```python
from build123d import *
from build123d.topology import SkipClean

# Parameters (mm, degrees)
EXTRUSION1_DEPTH = 20
ESQUISSE2_R      = 3.5
EXTRUSION2_DEPTH = 8
EXTRUSION3_START = -3
EXTRUSION3_DEPTH = 3


with BuildPart() as part:
    # Esquisse1 → Extrusion1 (new body)
    with BuildSketch(Plane.XY):
        Polygon((-21.808080808, -11.643556434), (-21.808080808, 14.356443566), (-28.808080808, 14.356443566), (-28.808080808, 16.356443566), (-21.808080808, 16.356443566), (-21.808080808, 23.356443566), (18.191919192, 23.356443566), (18.191919192, 16.356443566), (25.191919192, 16.356443566), (25.191919192, 14.356443566), (18.191919192, 14.356443566), (18.191919192, -11.643556434), align=None)
    extrude(amount=EXTRUSION1_DEPTH)

    # Esquisse2 → Extrusion2 (add)
    with BuildSketch(Plane(origin=(0, 23.356443566, 0), x_dir=(1, 0, 0), z_dir=(0, 1, 0))):
        with Locations((8.191919192, -10)):
            Circle(ESQUISSE2_R)
    extrude(amount=EXTRUSION2_DEPTH)

    # Esquisse3 → Extrusion3 (add)
    with SkipClean():  # the faces are left unmerged after this step: merging them gives an invalid solid
        with BuildSketch(Plane(origin=(0, 31.356443566, 0), x_dir=(1, 0, 0), z_dir=(0, 1, 0)).offset(EXTRUSION3_START)):
            with BuildLine():
                Line((4.746696028, -9.383203961), (-5.515585224, 0.879077291))
                ThreePointArc((-5.515585224, 0.879077291), (-4.182449479, 2.374368671), (-2.687158099, 3.707504416))
                Line((-2.687158099, 3.707504416), (7.575123153, -6.554776836))
                ThreePointArc((7.575123153, -6.554776836), (8.191919192, -6.5), (8.808715231, -6.554776836))
                Line((8.808715231, -6.554776836), (19.069778625, 3.706286557))
                ThreePointArc((19.069778625, 3.706286557), (20.565077985, 2.373158793), (21.898205749, 0.877859433))
                Line((21.898205749, 0.877859433), (11.637142355, -9.383203961))
                ThreePointArc((11.637142355, -9.383203961), (11.691919192, -10), (11.637142355, -10.616796039))
                Line((11.637142355, -10.616796039), (21.899423607, -20.879077291))
                ThreePointArc((21.899423607, -20.879077291), (20.566287863, -22.374368671), (19.070996483, -23.707504416))
                Line((19.070996483, -23.707504416), (8.808715231, -13.445223164))
                ThreePointArc((8.808715231, -13.445223164), (8.191919192, -13.5), (7.575123153, -13.445223164))
                Line((7.575123153, -13.445223164), (-2.687158099, -23.707504416))
                ThreePointArc((-2.687158099, -23.707504416), (-4.182449479, -22.374368671), (-5.515585224, -20.879077291))
                Line((-5.515585224, -20.879077291), (4.746696028, -10.616796039))
                ThreePointArc((4.746696028, -10.616796039), (4.691919192, -10), (4.746696028, -9.383203961))
            make_face()
        extrude(amount=EXTRUSION3_DEPTH)


solid = part.part
```
Can you work these out from the model? Positions are in its coordinate system, mm. A direction names the side the tool comes from. Round coordinates to 2 decimals unless told otherwise and drop trailing zeros. Loops run counter-clockwise (first coordinate to the right, second up) from the corner with the lowest first, then second, coordinate; pieces in that order, holes last. Notation, with made-up numbers: M -17,-18 L 39,-18 A27 ccw 39,1 Z; hole C -32,-24.75 d7. An arc over 180 degrees is marked long. Write item = value, one per line. Start each with the question number.
(1) If we mould it in two halves opening along Y, with no side actions, what happens to faces 1 (the face through (-0.456, 29.835, 15.82)), 2 (the face through (-2, -11.644, 10)), 3 (the face through (15, 28.356, 2)), 4 (the face through (1, 28.356, 3))? For each: released by +Y, released by -Y, zero draft, split by the parting line, or undercut.
(2) Suppose I cut it at B-B on y = 15.5. Write out the boundary of the cut face in (x, z), plus the area to 3 significant figures.
(3) Suppose I cut it at A-A on z = 15.5. Write out the boundary of the cut face in (x, y).
(4) Suppose I cut it at C-C on x = -12. Write out the boundary of the cut face in (y, z).
(5) I need wall thicknesses on line 1 along Y through (x, z) = (13.5, 15.75); line 2 along Y through (x, z) = (-12.5, 8.25); line 3 along Z through (x, y) = (6, 19). Which ranges of each line are inside material? Lowest first, please.
(6) I'm going to push flat-ended pins straight in: P1, Ø2, axis at x = 20, z = 13, coming from the -Y side; P2, Ø5, axis at x = -17.5, y = 4, coming from the -Z side; P3, Ø7.5, axis at y = 21, z = 6, coming from the +X side. Where does each tip first touch, or does it pass through?
(7) Which directions (+Z, -Z, +X, -X, +Y, -Y) give clear straight access to the entire face, cutting with the end or side of a thin tool? Please do faces 5 (the face through (13.867, 29.835, 1.496)), 6 (the face through (16.7, 29.84, 15.68)), 7 (the face through (-25, 16.356, 10)), 8 (the face through (18.192, 2, 10)).
Answer block:
q1.face_1 = zero draft
q1.face_2 = released by -Y
q1.face_3 = undercut
q1.face_4 = undercut
q2.outline = M -28.81,0 L 25.19,0 L 25.19,20 L -28.81,20 Z
q2.area = 1,080 mm²
q3.outline = M -28.81,14.36 L -21.81,14.36 L -21.81,-11.64 L 18.19,-11.64 L 18.19,14.36 L 25.19,14.36 L 25.19,16.36 L 18.19,16.36 L 18.19,23.36 L -21.81,23.36 L -21.81,16.36 L -28.81,16.36 Z; M -0.14,28.36 L 5.52,28.36 L 5.52,31.36 L -0.14,31.36 Z; M 10.86,28.36 L 16.52,28.36 L 16.52,31.36 L 10.86,31.36 Z
q4.outline = M -11.64,0 L 23.36,0 L 23.36,20 L -11.64,20 Z
q5.line_1 = -11.64 to 23.36, 28.36 to 31.36
q5.line_2 = -11.64 to 23.36
q5.line_3 = 0 to 20
q6.P1 = 14.36
q6.P2 = 0
q6.P3 = 18.19
q7.face_5 = -Z, +Y
q7.face_6 = +X, +Y
q7.face_7 = +Z, -Z, -X, +Y
q7.face_8 = +Z, -Z, +X, -Y
